The listing builds one solid part. Answer for the finished solid, in the listing's coordinates (mm). Face numbers are marked on the shaded views. A direction names the side the tool comes from. Round coordinates to 2 decimals unless told otherwise and drop trailing zeros. Write each loop counter-clockwise with the first axis right and the second up, starting at its lowest first coordinate (ties: lowest second). Pieces come first, ordered by that corner, then holes. Notation, with made-up numbers: M 72,76.25 L 110,76.25 A34 ccw 110,111.25 Z; hole C -8,77 d5. An arc over 180 degrees is marked long. Put each result on its own line as item: value. Start each with the question number.
```python
from build123d import *

# Parameters (mm, degrees)
BOSS_EXTRUDE1_DEPTH = 6


with BuildPart() as part:
    # Sketch2 → Boss-Extrude1 (new body)
    with BuildSketch(Plane(origin=(0, 0, 0), x_dir=(1, 0, 0), z_dir=(0, 1, 0))):
        with BuildLine():
            Line((-38.998907426, 19.146898027), (-2.998907426, -16.853101973))
            ThreePointArc((-2.998907426, -16.853101973), (-2.565361924, -19.0326824), (-4.413120989, -20.267315535))
            Line((-4.413120989, -20.267315535), (-7.413120989, -20.267315535))
            Line((-7.413120989, -20.267315535), (-7.413120989, -26.267315535))
            Line((-7.413120989, -26.267315535), (-17.413120989, -26.267315535))
            Line((-17.413120989, -26.267315535), (-17.413120989, -20.267315535))
            Line((-17.413120989, -20.267315535), (-29.413120989, -20.267315535))
            Line((-29.413120989, -20.267315535), (-29.413120989, -26.267315535))
            Line((-29.413120989, -26.267315535), (-39.413120989, -26.267315535))
            Line((-39.413120989, -26.267315535), (-39.413120989, -20.267315535))
            Line((-39.413120989, -20.267315535), (-42.413120989, -20.267315535))
            Line((-42.413120989, -20.267315535), (-42.413120989, -17.267315535))
            Line((-42.413120989, -17.267315535), (-48.413120989, -17.267315535))
            Line((-48.413120989, -17.267315535), (-48.413120989, -7.267315535))
            Line((-48.413120989, -7.267315535), (-42.413120989, -7.267315535))
            Line((-42.413120989, -7.267315535), (-42.413120989, 4.732684465))
            Line((-42.413120989, 4.732684465), (-48.413120989, 4.732684465))
            Line((-48.413120989, 4.732684465), (-48.413120989, 14.732684465))
            Line((-48.413120989, 14.732684465), (-42.413120989, 14.732684465))
            Line((-42.413120989, 14.732684465), (-42.413120989, 17.732684465))
            ThreePointArc((-42.413120989, 17.732684465), (-41.178487854, 19.58044353), (-38.998907426, 19.146898027))
        make_face()
    extrude(amount=BOSS_EXTRUDE1_DEPTH)


solid = part.part
```
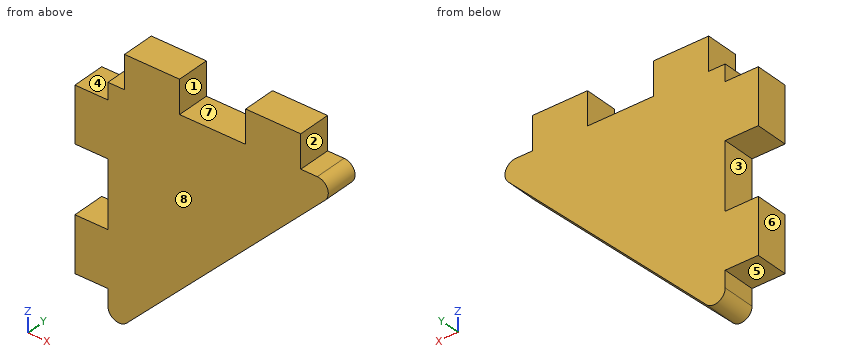
Item 1: Flat-ended cylindrical pins translate along their axes: pin 1 (3 mm diameter, centred on x = -46.5, y = 2.5, fed in from +Z); pin 2 (1.5 mm diameter, centred on y = 4.5, z = 8.5, fed in from +X); pin 3 (3.5 mm diameter, centred on y = 4, z = -17, fed in from -X); pin 4 (8 mm diameter, centred on x = -8.5, z = 2.5, fed in from +Y) (3 decimals). Find the tip coordinate at first contact, or state that the pin passes through.
Item 2: Section C-C (z = -16) is taken. Give the vertices of the cut face in (x, y).
Item 3: Determine the mould class of the marked faces 6, 7 and 8 for opening direction X: released by +X, released by -X, zero draft, split by the parting line, or undercut.
Item 4: Which of the six approach directions +Z, -Z, +X, -X, +Y, -Y give full straight-line access (tool end or side, diameter ignored) to the marked faces 1, 2, 3, 4 and 5?
Item 5: Consider line 1 along X through (y, z) = (4.8, 24); line 2 along Z through (x, y) = (-15.5, 3.2); line 3 along Z through (x, y) = (-8, 2.1). Determine where each line is inside the solid, lowest interval first. Write a range as [from, to].
Item 6: Section B-B (y = 3.55) is taken. Give the vertices of the cut face in (x, z), and give its area (3 significant figures).
Item 7: Section A-A (z = 21.5) is taken. Give the vertices of the cut face in (x, y).
Item 8: Section D-D (x = -13) is taken. Give the vertices of the cut face in (y, z).
Output values:
1. pin 1: stops at z = 17.27
1. pin 2: stops at x = -10.6
1. pin 3: stops at x = -42.41
1. pin 4: passes through
2. outline: M -42.41,0 L -35.85,0 L -35.85,6 L -42.41,6 Z
3. face 6: released by -X
3. face 7: undercut
3. face 8: zero draft
4. face 1: +Z, +Y, -Y
4. face 2: +Z, +X, +Y, -Y
4. face 3: -X, +Y, -Y
4. face 4: +Z, -X, +Y, -Y
4. face 5: -Z, -X, +Y, -Y
5. line 1: x = [-39.41, -29.41], [-17.41, -7.41]
5. line 2: z = [4.35, 26.27]
5. line 3: z = [11.85, 26.27]
6. outline: M -48.41,-14.73 L -42.41,-14.73 L -42.41,-17.73 A2 ccw -39,-19.15 L -3,16.85 A2 ccw -4.41,20.27 L -7.41,20.27 L -7.41,26.27 L -17.41,26.27 L -17.41,20.27 L -29.41,20.27 L -29.41,26.27 L -39.41,26.27 L -39.41,20.27 L -42.41,20.27 L -42.41,17.27 L -48.41,17.27 L -48.41,7.27 L -42.41,7.27 L -42.41,-4.73 L -48.41,-4.73 Z
6. area: 1,150 mm^2
7. outline: M -39.41,0 L -29.41,0 L -29.41,6 L -39.41,6 Z; M -17.41,0 L -7.41,0 L -7.41,6 L -17.41,6 Z
8. outline: M 0,6.85 L 6,6.85 L 6,26.27 L 0,26.27 Z
